Autodesk Inventor part; units mm, degrees
ref_plane "YZ Plane" through (0, 0, 0) normal (1, 0, 0) x (0, 1, 0)
ref_plane "XZ Plane" through (0, 0, 0) normal (0, 1, 0) x (-1, 0, 0)
ref_plane "XY Plane" through (0, 0, 0) normal (0, 0, 1) x (1, 0, 0)
sketch "Sketch1" plane through (0, 0, 0) normal (0, 0, 1) x (1, 0, 0)
  line L0 (17.2892, -53.3685) -> (9.2892, -53.3685)
  line L1 (-10.7108, -53.3685) -> (9.2892, -53.3685)
  line L2 (9.2892, 58.6315) -> (-10.7108, 38.6315)
  line L3 (17.2892, -53.3685) -> (17.2892, -49.7758)
  line L4 (17.2892, -46.9611) -> (17.2892, 27.2242)
  line L5 (17.2892, 30.0389) -> (17.2892, 41.6315)
  line L6 (17.2892, 41.6315) -> (17.2892, 51.5315)
  line L7 (17.2892, 63.6315) -> (17.2892, 56.6315)
  line L8 (9.2892, 63.6315) -> (17.2892, 63.6315) construction
  line L9 (17.2892, 63.6315) -> (9.5892, 63.6315)
  line L10 (9.5892, 63.6315) -> (9.5892, 59.3458)
  line L11 (9.2892, 58.6315) -> (9.2963, 58.6387)
  line L12 (9.2892, 60.6315) -> (9.2892, 63.6315) construction
  arc A0 (9.2963, 58.6387) -> (9.5892, 59.3458) centre (8.5892, 59.3458) ccw
  line L13 (17.2892, 27.2242) -> (17.2892, 30.0389)
  line L14 (17.2892, 51.5315) -> (17.2892, 56.6315)
  line L15 (17.2892, -49.7758) -> (17.2892, -46.9611)
  line L16 (-10.7108, -53.3685) -> (-12.7108, -53.3685)
  line L17 (-12.7108, -53.3685) -> (-12.7108, 36.6315)
  line L18 (-12.7108, 36.6315) -> (-10.7108, 38.6315)
  point P0 (0, 0)
  dimension "d2" = 0.3
  dimension "d3" = 1
  dimension "d19" = 30
extrude "Extrusion1" add sketch "Sketch1" along normal blind 3
ref_plane "Work Plane2" through (4.04, -8.0435, 0.345) normal (0, 0.7071, 0.7071) x (1, 0, 0)
sketch "Sketch3" plane through (4.04, -8.0435, 0.345) normal (0, 0.7071, 0.7071) x (1, 0, 0)
  line L0 (-4, 22) -> (-4, 0) construction
  line L1 (4, 22) -> (-4, 22) construction
  line L2 (4, 0) -> (4, 22) construction
  line L3 (-4, 0) -> (4, 0) construction
  line L4 (-5.5, 23.5) -> (-5.5, -1.5)
  line L5 (-5.5, 23.5) -> (5.5, 23.5)
  line L6 (5.5, 23.5) -> (5.5, -1.5)
  line L7 (5.5, -1.5) -> (-5.5, -1.5)
  point P0 (-4.04, 5.9315)
  dimension "d6" = 1.5
  dimension "d7" = 1.5
  dimension "d8" = 1.5
  dimension "d9" = 1.5
extrude "Extrusion2" cut sketch "Sketch3" along normal through all
sketch "Sketch4" plane through (0, 0, 3) normal (0, 0, 1) x (1, 0, 0)
  circle A0 centre (-5.7108, -43.3685) radius 2.25
  circle A1 centre (4.2892, -43.3685) radius 2.25
  circle A2 centre (-5.7108, 36.6315) radius 2.25
  circle A3 centre (4.2892, 36.6315) radius 2.25
  point P0 (0, 0)
hole "Hole1" at (-5.7108, -43.3685, 3) at (4.2892, -43.3685, 3) at (-5.7108, 36.6315, 3) at (4.2892, 36.6315, 3) direction (0, 0, -1) diameter 3.4 end through all countersink diameter 6.3 countersink angle 90
equation "\"d7\" = d6"
equation "\"d8\" = d6"
equation "\"d9\" = d6"
properties part number "BokPrawy"
Part model, mm, in its own coordinate system. A direction names the side the tool comes from. Coordinates: 2 decimals unless noted, no trailing zeros. Loops run counter-clockwise (first coordinate to the right, second up) from the corner with the lowest first, then second, coordinate; pieces in that order, holes last. Notation, with made-up numbers: M -10.5,20.25 L 17.5,20.25 A35 ccw 17.5,57.25 Z; hole C 3,59 d2. An arc over 180 degrees is marked long. Use a Markdown table: item, result. Add a question column.
Q1. Probe L1, parallel to X at y = 24.5, z = 2.2; L2, parallel to X at y = 37.5, z = 1.8; L3, parallel to Y at x = 9.5, z = 2.1. List the from-to ranges inside material, lowest first.
Q2. Pin check, flat tips, straight feed: P1, Ø1.5, axis at x = -5.5, z = 2.5, coming from the +Y side; P2, Ø0.9, axis at y = 61.5, z = 2, coming from the -X side; P3, Ø5.5, axis at x = -5.71, y = -43.37, coming from the +Z side; P4, Ø4, axis at x = 4.29, y = 36.63, coming from the -Z side. Stop position of each tip, or through.
Q3. Cut at B-B (z = 0.65). Give the number of separate pieces and of enclosed holes in the cut face, and give its area (3 significant figures).
Q4. Which spindle directions (+Z, -Z, +X, -X, +Y, -Y) get a long thin tool onto all of the face, cutting with end or side? Do faces 4 (the cylindrical face through (4.21, -41.67, 0.76)), 5 (the flat face through (9.589, 62, 1)), 6 (the flat face through (3.963, 26.325, 1.479)). Say none if no direction does.
Q5. Cut at A-A (x = 0). Write the cut outline in (y, z), and give its area (3 significant figures).
Q6. Mould opens along X. For faces 1 (the flat face through (2, -53.368, 1)), 2 (the flat face through (-12.711, -9, 1)), 3 (the cylindrical face through (3.78, 35.01, 0.76)) say: +X half, -X half, draft (parallel to the pull), parting line (faces both ways), or undercut.
Worked out:
| question | item | result |
|---|---|---|
| 1 | L1 | x = -12.71 to -1.46, 9.54 to 17.29 |
| 1 | L2 | x = -11.84 to -7.46, -3.96 to 2.54, 6.04 to 17.29 |
| 1 | L3 | y = -53.37 to -8.41, 26.95 to 58.93 |
| 2 | P1 | stops at y = 44.59 |
| 2 | P2 | stops at x = 9.59 |
| 2 | P3 | stops at z = 2.6 |
| 2 | P4 | stops at z = 0 |
| 3 | separate pieces | 1 |
| 3 | enclosed holes | 5 |
| 3 | area | 2,750 mm2 |
| 4 | face 4 | +Z, -Z |
| 4 | face 5 | +Z, -Z, -X, +Y |
| 4 | face 6 | +Z |
| 5 | outline | M -53.37,0 L -7.7,0 L -9.1,1.41 L -7.51,3 L -53.37,3 Z; M 24.85,0 L 49.34,0 L 49.34,3 L 27.85,3 Z |
| 5 | area | 204 mm2 |
| 6 | face 1 | draft |
| 6 | face 2 | -X half |
| 6 | face 3 | undercut |
